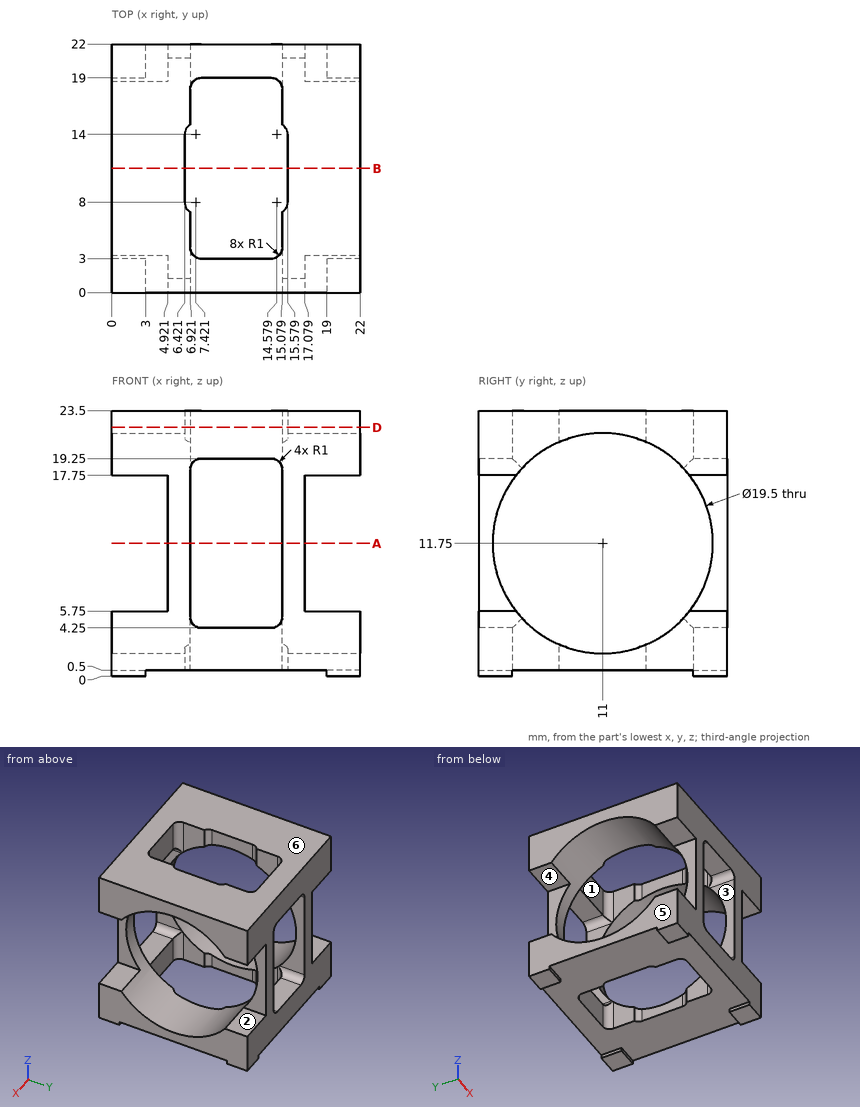
Study the drawing (mm; zero at the part's minimum x, y, z) and answer. A direction names the side the tool comes from. Give positions to 0.01 mm unless a question says otherwise; leave off trailing zeros. Write each loop counter-clockwise with the first axis right and the second up, starting at its lowest first coordinate (ties: lowest second). Pieces come first, ordered by that corner, then holes. Notation, with made-up numbers: M 47,19 L 84,19 A19 ccw 84,40 Z; hole C -1,39 d2. An arc over 180 degrees is marked long. Put each result on its own line as item: value. Start each with the question number.
1. Each of these flat-tipped pins is pushed along its axis until it touches: pin 1 Ø2.5 at (y, z) = (1, 12) entering from -X; pin 2 Ø3 at (x, z) = (8.5, 15) entering from +Y; pin 3 Ø4 at (y, z) = (2.5, 12) entering from +X; pin 4 Ø3.5 at (x, y) = (12, 1) entering from -Z. Where does it stop, or does it pass through?
2. The part is cut by section D-D, the plane z = 22. Give the vertices of the cut face in (x, y), and give its area (3 significant figures).
3. For a pull along Z with two mould halves and no side action, classify the marked faces 4, 5 and 6 as released by +Z, released by -Z, zero draft, split by the parting line, or undercut.
4. The part is cut by section A-A, the plane z = 11.75. Give the vertices of the cut face in (x, y), and give its area (3 significant figures).
5. The part is cut by section B-B, the plane y = 11. Give the vertices of the cut face in (x, z).
6. Which of the six approach directions +Z, -Z, +X, -X, +Y, -Y give full straight-line access (tool end or side, diameter ignored) to the marked faces 1, 2 and 3?
7. Consider line 1 along Y through (x, z) = (11.25, 22.25); line 2 along Y through (x, z) = (5.25, 11.75); line 3 along Z through (x, y) = (11, 20.25). Determine where each line is inside the solid, lowest interval first.
Final values:
1. pin 1: stops at x = 4.92
1. pin 2: passes through
1. pin 3: stops at x = 17.08
1. pin 4: stops at z = 0.5
2. outline: M 0,0 L 22,0 L 22,22 L 0,22 Z; hole M 6.42,8 A1 ccw 6.92,7.13 L 6.92,4 A1 ccw 7.92,3 L 14.08,3 A1 ccw 15.08,4 L 15.08,7.13 A1 ccw 15.58,8 L 15.58,14 A1 ccw 15.08,14.87 L 15.08,18 A1 ccw 14.08,19 L 7.92,19 A1 ccw 6.92,18 L 6.92,14.87 A1 ccw 6.42,14 Z
2. area: 347 mm²
3. face 4: undercut
3. face 5: zero draft
3. face 6: released by +Z
4. outline: M 4.92,0 L 6.92,0 L 6.92,1.25 L 4.92,1.25 Z; M 4.92,20.75 L 6.92,20.75 L 6.92,22 L 4.92,22 Z; M 15.08,0 L 17.08,0 L 17.08,1.25 L 15.08,1.25 Z; M 15.08,20.75 L 17.08,20.75 L 17.08,22 L 15.08,22 Z
4. area: 10.0 mm²
5. outline: M 0,0.5 L 6.42,0.5 L 6.42,2 L 0,2 Z; M 0,21.5 L 6.42,21.5 L 6.42,23.5 L 0,23.5 Z; M 15.58,0.5 L 22,0.5 L 22,2 L 15.58,2 Z; M 15.58,21.5 L 22,21.5 L 22,23.5 L 15.58,23.5 Z
6. face 1: +Z, -Z
6. face 2: +X, +Y, -Y
6. face 3: +Y, -Y
7. line 1: y = 0 to 3, 19 to 22
7. line 2: y = 0 to 1.25, 20.75 to 22
7. line 3: z = 0.5 to 4.25, 19.25 to 23.5
